```python
from build123d import *

# Parameters (mm, degrees)
F0_R          = 90
F0_R_2        = 25
F1_DEPTH      = 30
F0_R_3        = 7.5
F2_DEPTH      = 35
F3_R          = 14.99999
F4_DEPTH      = 5
F5_DEPTH      = 15
F5_DEPTH_BACK = 45


# Not quite as in the source:
# - a fillet or chamfer is up to 0.001 mm smaller than in the source, because OpenCascade refuses the exact size


with BuildPart() as f1:
    # F0 (on Front) → F1 (new body)
    with BuildSketch(Plane.XZ):
        Circle(F0_R)
        Circle(F0_R_2, mode=Mode.SUBTRACT)
    extrude(amount=F1_DEPTH)

    # F0 (on Front) → F2 (join)
    with BuildSketch(Plane.XZ):
        Circle(F0_R_2)
        Circle(F0_R_3, mode=Mode.SUBTRACT)
    extrude(amount=F2_DEPTH)

    # F3 (radius 15 in the source; OpenCascade refuses exactly that, so slightly less here)
    f3_edges = [f1.edges().sort_by_distance(p)[0] for p in [
        (-90, -30, 0),
        (-90, 0, 0),
    ]]
    fillet(f3_edges, radius=F3_R)

    # F0 (on Front) → F4 (join)
    with BuildSketch(Plane.XZ):
        Circle(F0_R_2)
        Circle(F0_R_3, mode=Mode.SUBTRACT)
    extrude(amount=-F4_DEPTH)

    # F0 (on Front) → F5 (join, two sides)
    with BuildSketch(Plane.XZ) as f5_sk:
        Circle(F0_R_3)
    extrude(amount=-F5_DEPTH)
    extrude(f5_sk.sketch, amount=F5_DEPTH_BACK)


solid = f1.part
```
The listing builds one solid part. Answer for the finished solid, in the listing's coordinates (mm). A direction names the side the tool comes from. Give positions to 0.01 mm unless a question says otherwise; leave off trailing zeros. Order: outer loops, then holes, each group sorted by start corner. A loop starts at its lowest first (then second) coordinate and runs counter-clockwise, first axis right, second up. Notation, with made-up numbers: (11.25, 53.25) -> (39.25, 53.25) arc R16 cw to (39.25, 68.25) -> close; hole circle Ø6 at (64.5, 46.5). An arc over 180 degrees is marked (long way). Answer as a JSON object with one key per item and string values. Group by question number.
Item 1: A tool of negligible diameter and unlimited length cuts with its end or side. For faces 1 (the flat face through (-6, -35, -5)), 2 (the cylindrical face through (-7.493, 9.93, 0.33)), 3 (the flat face through (0, -45, 0)), from which of +Z, -Z, +X, -X, +Y, -Y can it reach the whole face along a straight path? Write none if from no direction.
Item 2: Flat-ended cylindrical pins translate along their axes: pin 1 (12 mm diameter, centred on x = -3.5, z = 55, fed in from +Y); pin 2 (1 mm diameter, centred on x = -49.5, y = -4.5, fed in from -Z); pin 3 (1.5 mm diameter, centred on x = 37.5, y = 2.5, fed in from +Z); pin 4 (4 mm diameter, centred on y = -5, z = -13.5, fed in from -X). Find the tip coordinate at first contact, or state that the pin passes through.
Item 3: Consider L1, parallel to Y at x = 46.5, z = 43.5; L2, parallel to Y at x = 18.5, z = 5; L3, parallel to Z at x = 16, y = 4. Determine where each line is inside the solid, lowest interval first. Write a range as from..to.
Item 4: The part is cut by section D-D on y = -22. Write down the section's boundary in (x, z).
Item 5: The part is cut by section C-C on y = -11. Write down the section's boundary in (x, z), and give its area (3 significant figures).
Result set:
{
 "1": {"face 1": "-Y", "face 2": "+Y", "face 3": "+Z, -Z, +X, -X, -Y"},
 "2": {"pin 1": "y = 0", "pin 2": "z = -70.65", "pin 3": "through", "pin 4": "x = -86.68"},
 "3": {"L1": "-30..0", "L2": "-35..5", "L3": "-19.21..19.21"},
 "4": {"outline": "circle Ø176.53 at (0, 0)"},
 "5": {"outline": "circle Ø178.91 at (0, 0)", "area": "25,100 mm²"}
}
